The listing builds one solid part. Answer for the finished solid, in the listing's coordinates (mm). Face numbers are marked on the shaded views. Coordinates: 2 decimals unless noted, no trailing zeros. Order: outer loops, then holes, each group sorted by start corner. A loop starts at its lowest first (then second) coordinate and runs counter-clockwise, first axis right, second up. Notation, with made-up numbers: (-29, 27.25) -> (-21, 27.25) arc R32 cw to (-21, 61.25) -> close; hole circle Ø4 at (45.25, -13.75). An arc over 180 degrees is marked (long way). Write each question's results on one line, items separated by ' | '. Start each with the question number.
(1) The part is cut by section C-C, the plane z = -44.5. Give the vertices of the cut face in (x, y), then the cut area to 3 significant figures.
(2) The part is cut by section D-D, the plane x = -6. Give the vertices of the cut face in (y, z), then the cut area to 3 significant figures.
(3) Straight lines are drawn through the part: L1, parallel to Z at x = 26, y = 1.85; L2, parallel to X at y = 1.4, z = 11.5; L3, parallel to X at y = 3.65, z = 8. For each, find the intervals that lie inside material, in ascending order.
(4) Given pin 1 (1.5 mm diameter, centred on y = 3.5, z = -38.5, fed in from -X); pin 2 (2.5 mm diameter, centred on x = -26, z = -48.5, fed in from -Y); pin 3 (4.5 mm diameter, centred on x = 26, z = 11.5, fed in from +Y); pin 4 (0.9 mm diameter, centred on x = 5.5, y = 3, fed in from +Z), each flat-ended and moving along its own axis, determine where each tip first touches the part or whether it passes through.
(5) The part is cut by section A-A, the plane x = -26. Count the separate pieces of the cut face and the enclosed holes in it, then the cut area to 3 significant figures.
(6) Determine the mould class of the marked faces 1 and 2 for opening direction Z: +Z half, -Z half, draft (parallel to the pull), parting line (faces both ways), or undercut.
(7) The part is cut by section B-B, the plane z = -23.5. Give the vertices of the cut face in (x, y), then the cut area to 3 significant figures.
```python
from build123d import *

# Parameters (mm, degrees)
SKETCH1_W           = 64
SKETCH1_H           = 109
BOSS_EXTRUDE1_DEPTH = 2
SKETCH2_W           = 60
SKETCH2_H           = 105
BOSS_EXTRUDE2_DEPTH = 3
SKETCH3_W           = 58
SKETCH3_H           = 103
CUT_EXTRUDE1_DEPTH  = 3
SKETCH4_R           = 1.5
CUT_EXTRUDE2_DEPTH  = 2
SKETCH6_R           = 2.5
CUT_EXTRUDE3_DEPTH  = 1
SKETCH7_R           = 2.45
CUT_EXTRUDE4_DEPTH  = 2
SKETCH8_W           = 8
SKETCH8_H           = 13
CUT_EXTRUDE5_DEPTH  = 2
SKETCH9_W           = 8
SKETCH9_H           = 13
CUT_EXTRUDE6_DEPTH  = 2
FILLET2_R           = 1
FILLET3_R           = 1
FILLET4_R           = 2
FILLET5_R           = 2
FILLET6_R           = 1
SKETCH10_W          = 8
SKETCH10_H          = 17
CUT_EXTRUDE7_DEPTH  = 1
SKETCH11_R          = 0.75
CUT_EXTRUDE8_DEPTH  = 2


with BuildPart() as part:
    # Sketch1 → Boss-Extrude1 (new body)
    with BuildSketch(Plane(origin=(0, 0, 0), x_dir=(1, 0, 0), z_dir=(0, 1, 0))):
        Rectangle(SKETCH1_W, SKETCH1_H)
    extrude(amount=BOSS_EXTRUDE1_DEPTH)

    # Sketch2 → Boss-Extrude2 (add)
    with BuildSketch(Plane(origin=(0, 2, 0), x_dir=(1, 0, 0), z_dir=(0, 1, 0))):
        Rectangle(SKETCH2_W, SKETCH2_H)
    extrude(amount=BOSS_EXTRUDE2_DEPTH)

    # Sketch3 → Cut-Extrude1 (cut)
    with BuildSketch(Plane(origin=(0, 5, 0), x_dir=(1, 0, 0), z_dir=(0, 1, 0))):
        Rectangle(SKETCH3_W, SKETCH3_H)
    extrude(amount=-CUT_EXTRUDE1_DEPTH, mode=Mode.SUBTRACT)

    # Sketch4 → Cut-Extrude2 (cut)
    with BuildSketch(Plane(origin=(0, 2, 0), x_dir=(1, 0, 0), z_dir=(0, 1, 0))):
        with Locations(Location((-26, 48.5, 0), (0, 0, 270))):
            Circle(SKETCH4_R)
        with Locations(Location((-26, -11.5, 0), (0, 0, 270))):
            Circle(SKETCH4_R)
        with Locations(Location((26, -11.5, 0), (0, 0, 90))):
            Circle(SKETCH4_R)
        with Locations(Location((26, 48.5, 0), (0, 0, 90))):
            Circle(SKETCH4_R)
    extrude(amount=-CUT_EXTRUDE2_DEPTH, mode=Mode.SUBTRACT)

    # Sketch6 → Cut-Extrude3 (cut)
    with BuildSketch(Plane.XZ):
        with Locations(Location((26, -48.5, 0), (0, 0, 270))):
            Circle(SKETCH6_R)
        with Locations(Location((-26, -48.5, 0), (0, 0, 270))):
            Circle(SKETCH6_R)
        with Locations(Location((26, 11.5, 0), (0, 0, 270))):
            Circle(SKETCH6_R)
        with Locations(Location((-26, 11.5, 0), (0, 0, 270))):
            Circle(SKETCH6_R)
    extrude(amount=-CUT_EXTRUDE3_DEPTH, mode=Mode.SUBTRACT)

    # Sketch7 → Cut-Extrude4 (cut)
    with BuildSketch(Plane(origin=(0, 2, 0), x_dir=(1, 0, 0), z_dir=(0, 1, 0))):
        with Locations(Location((0, 44.5, 0), (0, 0, 270))):
            Circle(SKETCH7_R)
    extrude(amount=-CUT_EXTRUDE4_DEPTH, mode=Mode.SUBTRACT)

    # Sketch8 → Cut-Extrude5 (cut)
    with BuildSketch(Plane(origin=(0, 2, 0), x_dir=(1, 0, 0), z_dir=(0, 1, 0))):
        with Locations((-15, 23)):
            Rectangle(SKETCH8_W, SKETCH8_H)
    extrude(amount=-CUT_EXTRUDE5_DEPTH, mode=Mode.SUBTRACT)

    # Sketch9 → Cut-Extrude6 (cut)
    with BuildSketch(Plane(origin=(0, 2, 0), x_dir=(1, 0, 0), z_dir=(0, 1, 0))):
        with Locations((15, 23)):
            Rectangle(SKETCH9_W, SKETCH9_H)
    extrude(amount=-CUT_EXTRUDE6_DEPTH, mode=Mode.SUBTRACT)

    # Fillet2
    fillet2_edges = [part.edges().sort_by_distance(p)[0] for p in [
        (32, 1, -54.5),
    ]]
    fillet(fillet2_edges, radius=FILLET2_R)

    # Fillet3
    fillet3_edges = [part.edges().sort_by_distance(p)[0] for p in [
        (-32, 1, -54.5),
    ]]
    fillet(fillet3_edges, radius=FILLET3_R)

    # Fillet4
    fillet4_edges = [part.edges().sort_by_distance(p)[0] for p in [
        (-32, 1, 54.5),
    ]]
    fillet(fillet4_edges, radius=FILLET4_R)

    # Fillet5
    fillet5_edges = [part.edges().sort_by_distance(p)[0] for p in [
        (32, 1, 54.5),
    ]]
    fillet(fillet5_edges, radius=FILLET5_R)

    # Fillet6
    fillet6_edges = [part.edges().sort_by_distance(p)[0] for p in [
        (0, 0, -54.5),
        (31.707106781, 0, -54.207106781),
        (-32, 0, -0.5),
        (-31.707106781, 0, -54.207106781),
        (0, 0, 54.5),
        (-31.414213562, 0, 53.914213562),
        (32, 0, -0.5),
        (31.414213562, 0, 53.914213562),
    ]]
    fillet(fillet6_edges, radius=FILLET6_R)

    # Sketch10 → Cut-Extrude7 (cut)
    with BuildSketch(Plane(origin=(0, 2, 0), x_dir=(1, 0, 0), z_dir=(0, 1, 0))):
        with Locations((-15, 23)):
            Rectangle(SKETCH10_W, SKETCH10_H)
        with Locations((15, 23)):
            Rectangle(SKETCH10_W, SKETCH10_H)
    extrude(amount=-CUT_EXTRUDE7_DEPTH, mode=Mode.SUBTRACT)

    # Sketch11 → Cut-Extrude8 (cut)
    with BuildSketch(Plane(origin=(0, 2, 0), x_dir=(1, 0, 0), z_dir=(0, 1, 0))):
        with Locations(Location((0, -11.5, 0), (0, 0, 270))):
            Circle(SKETCH11_R)
        with Locations(Location((0, -9, 0), (0, 0, 270))):
            Circle(SKETCH11_R)
        with Locations(Location((1.767766953, -9.732233047, 0), (0, 0, 270))):
            Circle(SKETCH11_R)
        with Locations(Location((2.5, -11.5, 0), (0, 0, 270))):
            Circle(SKETCH11_R)
        with Locations(Location((1.767766953, -13.267766953, 0), (0, 0, 270))):
            Circle(SKETCH11_R)
        with Locations(Location((0, -14, 0), (0, 0, 270))):
            Circle(SKETCH11_R)
        with Locations(Location((-1.767766953, -9.732233047, 0), (0, 0, 270))):
            Circle(SKETCH11_R)
        with Locations(Location((-2.5, -11.5, 0), (0, 0, 270))):
            Circle(SKETCH11_R)
        with Locations(Location((-1.767766953, -13.267766953, 0), (0, 0, 270))):
            Circle(SKETCH11_R)
    extrude(amount=-CUT_EXTRUDE8_DEPTH, mode=Mode.SUBTRACT)


solid = part.part
```
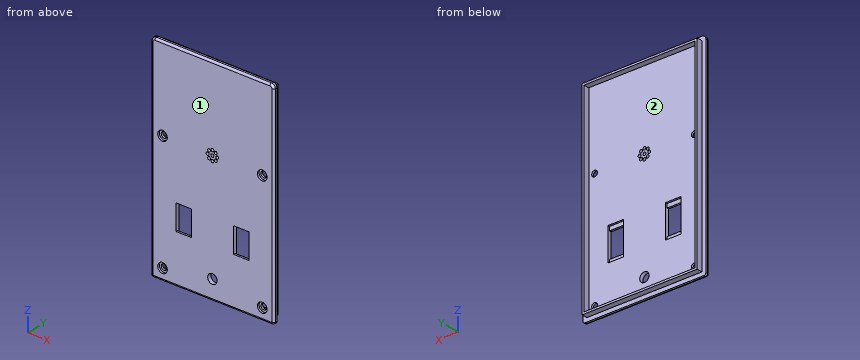
Established:
1) outline: (-32, 1) arc R1 ccw to (-31, 0) -> (-2.45, 0) -> (-2.45, 2) -> (-29, 2) -> (-29, 5) -> (-30, 5) -> (-30, 2) -> (-32, 2) -> close; (2.45, 0) -> (31, 0) arc R1 ccw to (32, 1) -> (32, 2) -> (30, 2) -> (30, 5) -> (29, 5) -> (29, 2) -> (2.45, 2) -> close | area: 124 mm^2
2) outline: (0, -53.5) arc R1 ccw to (1, -54.5) -> (2, -54.5) -> (2, -52.5) -> (5, -52.5) -> (5, -51.5) -> (2, -51.5) -> (2, 51.5) -> (5, 51.5) -> (5, 52.5) -> (2, 52.5) -> (2, 54.5) -> (1, 54.5) arc R1 ccw to (0, 53.5) -> close | area: 224 mm^2
3) L1: z = -54.5 to -50, -47 to 10, 13 to 54.5 | L2: x = -32 to -27.5, -24.5 to -3.25, -1.75 to -0.75, 0.75 to 1.75, 3.25 to 24.5, 27.5 to 32 | L3: x = -30 to -29, 29 to 30
4) pin 1: stops at x = -30 | pin 2: passes through | pin 3: stops at y = 2 | pin 4: stops at z = 52.5
5) separate pieces: 3 | enclosed holes: 0 | area: 208 mm^2
6) face 1: draft | face 2: undercut
7) outline: (-32, 1) arc R1 ccw to (-31, 0) -> (-19, 0) -> (-19, 2) -> (-29, 2) -> (-29, 5) -> (-30, 5) -> (-30, 2) -> (-32, 2) -> close; (-11, 0) -> (11, 0) -> (11, 2) -> (-11, 2) -> close; (19, 0) -> (31, 0) arc R1 ccw to (32, 1) -> (32, 2) -> (30, 2) -> (30, 5) -> (29, 5) -> (29, 2) -> (19, 2) -> close | area: 102 mm^2
